Autodesk Inventor part; units mm, degrees
ref_plane "YZ Plane" through (0, 0, 0) normal (1, 0, 0) x (0, 1, 0)
ref_plane "XZ Plane" through (0, 0, 0) normal (0, 1, 0) x (-1, 0, 0)
ref_plane "XY Plane" through (0, 0, 0) normal (0, 0, 1) x (1, 0, 0)
sketch "Sketch5" plane through (0, 0, 0) normal (0, 0, 1) x (1, 0, 0)
  line L0 (-22, 43) -> (22, 43)
  line L1 (22, 43) -> (22, -43)
  line L2 (22, -43) -> (-22, -43)
  line L3 (-22, -43) -> (-22, 43)
  point P0 (0, 0)
  point P1 (22, 0)
  point P2 (0, 43)
  dimension "d8" = 86
  dimension "d9" = 44
extrude "Extrusion5" add sketch "Sketch5" along normal mid plane 107.5
sketch "Sketch6" plane through (0, 0, 53.75) normal (0, 0, 1) x (1, 0, 0)
  line L0 (22, 43) -> (-22, 43)
  circle A0 centre (14, -33) radius 4
  circle A1 centre (-14, -33) radius 4
  circle A2 centre (-14, -33) radius 8.5
  point P0 (0, 0)
  dimension "d12" = 76
  dimension "d13" = 28
  dimension "d14" = 14
  dimension "d15" = 8
  dimension "d17" = 17
hole "Hole1" at (-14, -33, 53.75) at (14, -33, 53.75) direction (0, 0, -1) diameter 8.5 end through all counterbore diameter 14 counterbore depth 45
sketch "Sketch7" plane through (22, -43, 53.75) normal (1, 0, 0) x (0, 0, -1)
  line L0 (0, 86) -> (107.5, 86)
  circle A0 centre (18.75, 78) radius 3
  circle A1 centre (88.75, 78) radius 3
  point P0 (53.75, 43)
  dimension "d25" = 8
  dimension "d26" = 70
  dimension "d27" = 35
  dimension "d28" = 6
  dimension "d45" = 107.5
  dimension "d46" = 18.75
hole "Hole2" at (22, 35, 35) at (22, 35, -35) direction (-1, 0, 0) diameter 4.917 end through all
sketch "Sketch8" plane through (0, 0, 53.75) normal (0, 0, 1) x (1, 0, 0)
  circle A0 centre (-14, -33) radius 7
  circle A1 centre (14, -33) radius 7
  line L0 (22, 43) -> (-22, 43)
  circle A2 centre (14, 28) radius 4
  circle A3 centre (-14, 28) radius 4
  point P0 (0, 0)
  dimension "d36" = 15
  dimension "d37" = 8
hole "Hole3" at (-14, 28, 53.75) at (14, 28, 53.75) direction (0, 0, -1) diameter 4.134 depth 15 tip angle 118
properties part number "BC-10015" material "Alumínio 7075"
Read the model definition and answer for the solid it produces. Units are mm, in the model's axes. A direction names the side the tool comes from. Give positions to 0.01 mm unless a question says otherwise; leave off trailing zeros. Order: outer loops, then holes, each group sorted by start corner. A loop starts at its lowest first (then second) coordinate and runs counter-clockwise, first axis right, second up. Notation, with made-up numbers: (-19.75, 53) -> (31.25, 53) arc R25 ccw to (31.25, 75) -> close; hole circle Ø4 at (54, 55.5). An arc over 180 degrees is marked (long way). Write item = value, one per line.
1. A cutting plane is placed at B-B, the plane y = -33. Write down the section's boundary in (x, z).
Numbers:
outline = (-22, -53.75) -> (-18.25, -53.75) -> (-18.25, 8.75) -> (-21, 8.75) -> (-21, 53.75) -> (-22, 53.75) -> close; (-9.75, -53.75) -> (9.75, -53.75) -> (9.75, 8.75) -> (7, 8.75) -> (7, 53.75) -> (-7, 53.75) -> (-7, 8.75) -> (-9.75, 8.75) -> close; (18.25, -53.75) -> (22, -53.75) -> (22, 53.75) -> (21, 53.75) -> (21, 8.75) -> (18.25, 8.75) -> close
2. Given pin 1 (11 mm diameter, centred on x = -14, y = -33, fed in from +Z); pin 2 (3.5 mm diameter, centred on x = -14, y = 28, fed in from +Z), each flat-ended and moving along its own axis, determine where each tip first touches the part or whether it passes through.
Numbers:
pin_1 = 8.75
pin_2 = 38.56
3. A cutting plane is placed at A-A, the plane z = 35. Write down the section's boundary in (x, y).
Numbers:
outline = (-22, -43) -> (22, -43) -> (22, 32.54) -> (-22, 32.54) -> close; (-22, 37.46) -> (22, 37.46) -> (22, 43) -> (-22, 43) -> close; hole circle Ø14 at (-14, -33); hole circle Ø14 at (14, -33)
4. The mould has two halves that part along Y. Classify faces 1 (the face through (0, -43, -1)), 2 (the face through (-0.31, 35.94, -37.27)), 3 (the face through (0, 1, 53.75)): +Y half, -Y half, draft (parallel to the pull), parting line (faces both ways), or undercut.
Numbers:
face_1 = -Y half
face_2 = undercut
face_3 = draft
5. A cutting plane is placed at D-D, the plane z = -44. Write down the section's boundary in (x, y).
Numbers:
outline = (-22, -43) -> (22, -43) -> (22, 43) -> (-22, 43) -> close; hole circle Ø8.5 at (-14, -33); hole circle Ø8.5 at (14, -33)
6. Straight lines are drawn through the part: line 1 along Y through (x, z) = (-14, 43); line 2 along X through (y, z) = (-33, 12.5); line 3 along X through (y, z) = (-33, -28.5). For each, find the intervals that lie inside material, in ascending order.
Numbers:
line_1 = -43 to -40, -26 to 25.93, 30.07 to 43
line_2 = -22 to -21, -7 to 7, 21 to 22
line_3 = -22 to -18.25, -9.75 to 9.75, 18.25 to 22
7. For faces 4 (the face through (0, 1, -53.75)), 5 (the face through (-14.62, 26.03, 46.14)), determine the directions among +Z, -Z, +X, -X, +Y, -Y from which every point of the face is accessible in a straight line to the end or side of a thin tool.
Numbers:
face_4 = -Z, +X, -X, +Y, -Y
face_5 = +Z
8. A cutting plane is placed at C-C, the plane z = 24. Write down the section's boundary in (x, y), and give its area (3 significant figures).
Numbers:
outline = (-22, -43) -> (22, -43) -> (22, 43) -> (-22, 43) -> close; hole circle Ø14 at (-14, -33); hole circle Ø14 at (14, -33)
area = 3,480 mm²
